Source: three-view drawing plus pictorial views. Frame: mm from the lowest corner of the part. A direction names the side the tool comes from. Give positions to 0.01 mm unless a question says otherwise; leave off trailing zeros. Write each loop counter-clockwise with the first axis right and the second up, starting at its lowest first coordinate (ties: lowest second). Pieces come first, ordered by that corner, then holes. Notation, with made-up numbers: (-18.5, 86) -> (1.5, 86) arc R23 cw to (1.5, 96) -> close; hole circle Ø9 at (-4, 45). An arc over 180 degrees is marked (long way). Answer in a Markdown table with one row per item. Add a question column.
Item 1: First-contact query: P1, Ø3.5, axis at x = 5, z = 12, coming from the -Y side; P2, Ø4, axis at x = 25.5, y = 12, coming from the -Z side; P3, Ø1, axis at y = 12.5, z = 6.5, coming from the +X side. Flat tips, straight axial feed; report the tip coordinate or a pass-through.
Item 2: Section query D-D on z = 13. Output: boundary loops of the cut face in (x, y).
Item 3: Section query A-A on z = 4. Output: boundary loops of the cut face in (x, y), plus the area to 3 significant figures.
Item 4: Section query C-C on y = 12. Output: boundary loops of the cut face in (x, z), plus the area to 3 significant figures.
Item 5: Access query for the marked faces 1, 2, 3 and 4. Directions: +Z, -Z, +X, -X, +Y, -Y. A direction counts if a zero-diameter tool reaches every point of the face in a straight line with its end or side. Return the directions, or none.
Item 6: Section query B-B on x = 15.5. Output: boundary loops of the cut face in (y, z), plus the area to 3 significant figures.
Item 7: Material intervals for probe 1 along Z at (x, y) = (12.75, 11.5) (1 decimal); probe 2 along X at (y, z) = (7.25, 17.5); probe 3 along X at (y, z) = (15.25, 36), sorted ascending. Write a range as from..to.
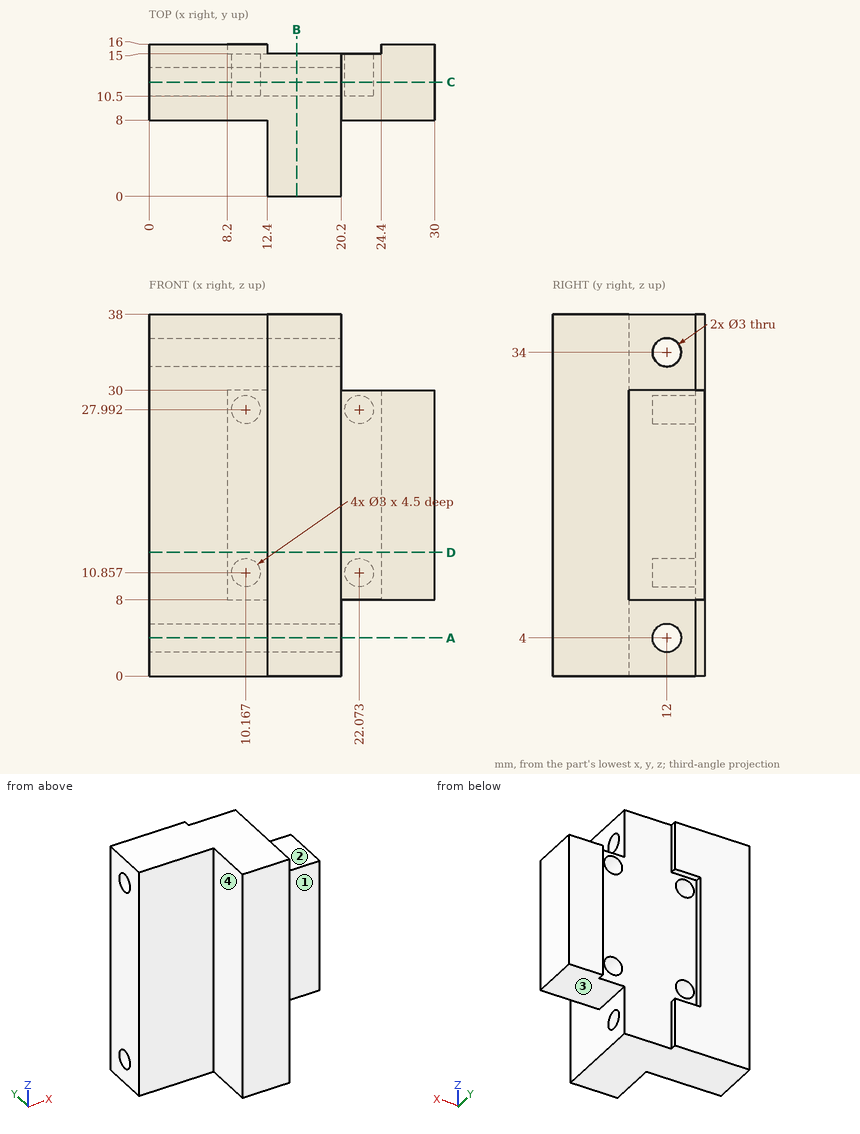
Findings below:
| question | item | result |
|---|---|---|
| 1 | P1 | stops at y = 8 |
| 1 | P2 | stops at z = 8 |
| 1 | P3 | stops at x = 20.2 |
| 2 | outline | (0, 8) -> (12.4, 8) -> (12.4, 0) -> (20.2, 0) -> (20.2, 8) -> (30, 8) -> (30, 16) -> (24.4, 16) -> (24.4, 15) -> (8.2, 15) -> (8.2, 16) -> (0, 16) -> close |
| 3 | outline | (0, 8) -> (12.4, 8) -> (12.4, 0) -> (20.2, 0) -> (20.2, 10.5) -> (0, 10.5) -> close; (0, 13.5) -> (20.2, 13.5) -> (20.2, 15) -> (12.4, 15) -> (12.4, 16) -> (0, 16) -> close |
| 3 | area | 156 mm^2 |
| 4 | outline | (0, 0) -> (20.2, 0) -> (20.2, 2.5) -> (0, 2.5) -> close; (0, 5.5) -> (20.2, 5.5) -> (20.2, 8) -> (30, 8) -> (30, 30) -> (20.2, 30) -> (20.2, 32.5) -> (0, 32.5) -> close; (0, 35.5) -> (20.2, 35.5) -> (20.2, 38) -> (0, 38) -> close; hole circle Ø3 at (10.17, 10.86); hole circle Ø3 at (10.17, 27.99); hole circle Ø3 at (22.07, 10.86); hole circle Ø3 at (22.07, 27.99) |
| 4 | area | 834 mm^2 |
| 5 | face 1 | +Z, -Z, +X, -Y |
| 5 | face 2 | +Z, +X, +Y, -Y |
| 5 | face 3 | -Z, +X, +Y, -Y |
| 5 | face 4 | +Z, -Z, -X, -Y |
| 6 | outline | (0, 0) -> (15, 0) -> (15, 38) -> (0, 38) -> close; hole circle Ø3 at (12, 4); hole circle Ø3 at (12, 34) |
| 6 | area | 556 mm^2 |
| 7 | probe 1 | z = 0..2.6, 5.4..32.6, 35.4..38 |
| 7 | probe 2 | x = 12.4..20.2 |
| 7 | probe 3 | x = 0..12.4 |
